```python
from build123d import *

# Parameters (mm, degrees)
SKETCH_1_W          = 15
SKETCH_1_H          = 15
SKETCH_1_W_2        = 13
SKETCH_1_H_2        = 13
EXTRUDE_1_DEPTH     = 180
SKETCH_2_R          = 2.5
SKETCH_2_R_2        = 1.5
CUT_EXTRUDE_1_DEPTH = 181.779561898
SKETCH_3_R          = 1.5
CUT_EXTRUDE_2_DEPTH = 181.779561898


with BuildPart() as part:
    # 草图1 → 凸台-拉伸1 (new body)
    with BuildSketch(Plane(origin=(0, 0, 0), x_dir=(1, 0, 0), z_dir=(0, 1, 0))):
        Rectangle(SKETCH_1_W, SKETCH_1_H)
        Rectangle(SKETCH_1_W_2, SKETCH_1_H_2, mode=Mode.SUBTRACT)
    extrude(amount=EXTRUDE_1_DEPTH)

    # 草图2 → 切除-拉伸1 (cut, through all)
    with BuildSketch(Plane.XY.offset(7.5)):
        with Locations((0, 134.901280605)):
            Circle(SKETCH_2_R)
        with Locations((0, 45.098719395)):
            Circle(SKETCH_2_R)
        with Locations((0, 187.5)):
            Circle(SKETCH_2_R_2)
        with Locations((0, 157.5)):
            Circle(SKETCH_2_R_2)
        with Locations((0, -7.5)):
            Circle(SKETCH_2_R_2)
        with Locations((0, 22.5)):
            Circle(SKETCH_2_R_2)
        with Locations((0, 105)):
            Circle(SKETCH_2_R_2)
        with Locations((0, 75)):
            Circle(SKETCH_2_R_2)
    extrude(amount=-CUT_EXTRUDE_1_DEPTH, mode=Mode.SUBTRACT)

    # 草图3 → 切除-拉伸2 (cut, through all)
    with BuildSketch(Plane(origin=(7.5, 0, 0), x_dir=(0, 0, -1), z_dir=(1, 0, 0))):
        with Locations((0, 170)):
            Circle(SKETCH_3_R)
        with Locations((0, 140)):
            Circle(SKETCH_3_R)
        with Locations(Location((0, 10, 0), (0, 0, 180))):
            Circle(SKETCH_3_R)
        with Locations(Location((0, 40, 0), (0, 0, 180))):
            Circle(SKETCH_3_R)
        Polygon((7.5, 172), (7.5, 180), (-0.5, 180), align=None)
        Polygon((-0.5, 0), (7.5, 8), (7.5, 0), align=None)
    extrude(amount=-CUT_EXTRUDE_2_DEPTH, mode=Mode.SUBTRACT)


solid = part.part
```
The model under review builds one solid part; all positions refer to its coordinate system, in mm. A direction names the side the tool comes from. Coordinates: 2 decimals unless noted, no trailing zeros. Loops run counter-clockwise (first coordinate to the right, second up) from the corner with the lowest first, then second, coordinate; pieces in that order, holes last. Notation, with made-up numbers: (28, -7) -> (40, -7) arc R20 cw to (40, 22) -> close; hole circle Ø11 at (42.5, -23). An arc over 180 degrees is marked (long way). Answer as CSV lines item,"result".
Item 1: For L1, parallel to X at y = 163.5, z = 4.75; L2, parallel to Z at x = 7.35, y = 170, list the stretches that pass through material, from the lowest coordinate up.
Results below:
L1,"x = -7.5 to -6.5, 6.5 to 7.5"
L2,"z = -7.5 to -1.5, 1.5 to 7.5"
Item 2: Take a section at D-D, the plane z = 3. State the section outline as (x, y) points.
Results below:
outline,"(-7.5, 0) -> (-6.5, 0) -> (-6.5, 180) -> (-7.5, 180) -> close; (6.5, 0) -> (7.5, 0) -> (7.5, 180) -> (6.5, 180) -> close"
Item 3: Draft analysis for pull direction Z (two halves, no side actions). For faces 1 (the flat face through (0, 89, -7.5)), 2 (the cylindrical face through (-0.542, 42.658, 7.007)), 3 (the cylindrical face through (-6.993, 11.464, -0.325)), state which applies: +Z half, -Z half, draft (parallel to the pull), parting line (faces both ways), or undercut.
Results below:
face 1,"-Z half"
face 2,"draft"
face 3,"undercut"
Item 4: Take a section at A-A, the plane y = 170. State the section outline as (x, z) points.
Results below:
outline,"(-7.5, -7.5) -> (7.5, -7.5) -> (7.5, -1.5) -> (6.5, -1.5) -> (6.5, -6.5) -> (-6.5, -6.5) -> (-6.5, -1.5) -> (-7.5, -1.5) -> close; (-7.5, 1.5) -> (-6.5, 1.5) -> (-6.5, 6.5) -> (6.5, 6.5) -> (6.5, 1.5) -> (7.5, 1.5) -> (7.5, 7.5) -> (-7.5, 7.5) -> close"
Item 5: Machinability: for faces 4 (the flat face through (-6.5, 89, 0)), 5 (the cylindrical face through (-0.195, 106.487, -6.993)), which of the approach directions +Z, -Z, +X, -X, +Y, -Y give a long, thin tool a straight path to every point of the face, cutting with its end or side? Answer none if there is none.
Results below:
face 4,"+Y, -Y"
face 5,"+Z, -Z"
Item 6: Take a section at B-B, the plane z = -3.5. State the section outline as (x, y) points, and give its area (3 significant figures).
Results below:
outline,"(-7.5, 4) -> (-6.5, 4) -> (-6.5, 176) -> (-7.5, 176) -> close; (6.5, 4) -> (7.5, 4) -> (7.5, 176) -> (6.5, 176) -> close"
area,"344 mm2"
Item 7: Take a section at C-C, the plane x = 0. Count the separate pieces of the cut face and the enclosed holes in it, and give its area (3 significant figures).
Results below:
separate pieces,"14"
enclosed holes,"0"
area,"301 mm2"
Item 8: Insertion check: pin 1 (4 mm diameter, centred on x = 0, y = 134.9, fed in from -Z). The pin has a flat end and moves straight along its axis. Give the tip position at first contact, or say it passes through.
Results below:
pin 1,"passes through"
